Verification items for this drawing (mm, ordinates from the low corner). A direction names the side the tool comes from. Coordinates: 2 decimals unless noted, no trailing zeros. Write each loop counter-clockwise with the first axis right and the second up, starting at its lowest first coordinate (ties: lowest second). Pieces come first, ordered by that corner, then holes. Notation, with made-up numbers: (-7.5, 54) -> (51.5, 54) arc R15 cw to (51.5, 61) -> close; hole circle Ø7 at (74.25, 14). An arc over 180 degrees is marked (long way). One line per question, with ' | ' between items.
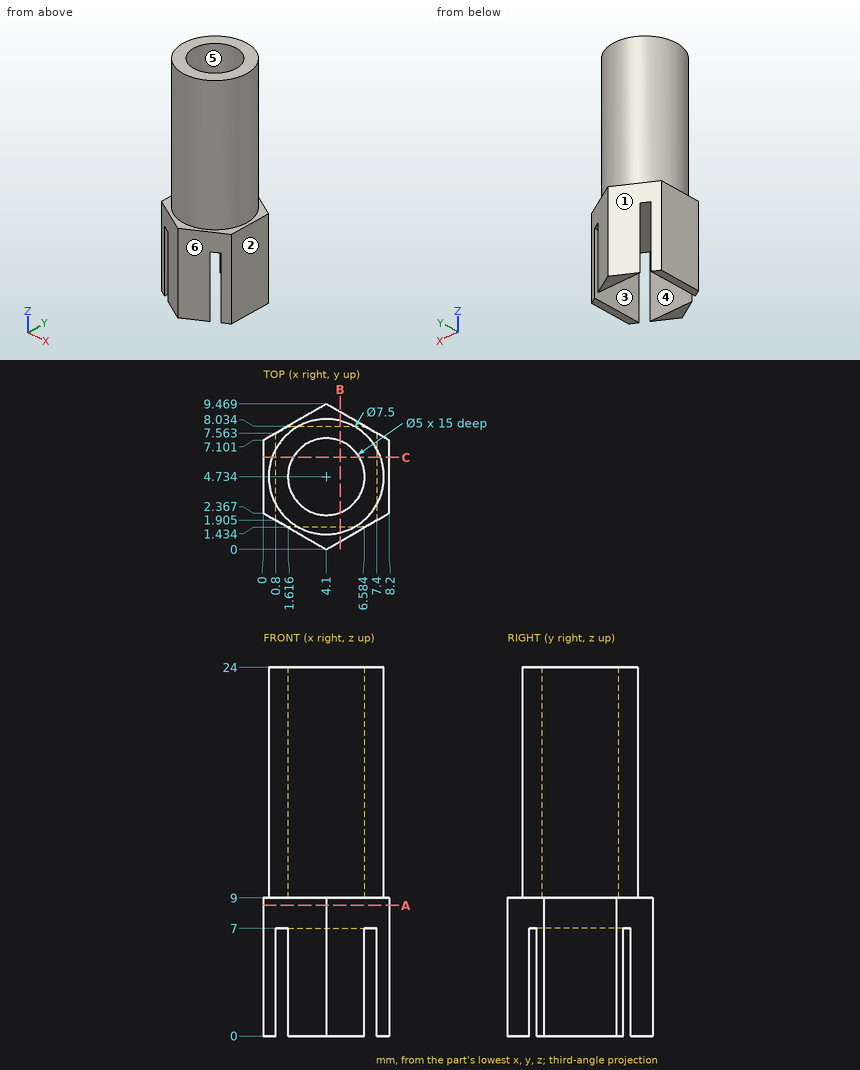
(1) Depth check by flat-ended pin: P1, Ø4, axis at y = 5.5, z = 11.5, coming from the +X side; P2, Ø1, axis at x = 5.5, y = 4, coming from the +Z side; P3, Ø3, axis at y = 8.5, z = 20, coming from the -X side; P4, Ø4, axis at x = 3, z = 4.5, coming from the +Y side. Enter the tip coordinate at first touch or a pass-through.
Answers below:
P1: stops at x = 7.85 | P2: stops at z = 9 | P3: stops at x = 1.11 | P4: stops at y = 9.47
(2) Material ranges on line 1 (Y direction, x = 4.1, z = 16) (1 decimal); line 2 (X direction, y = 4.75, z = 5.25); line 3 (Z direction, x = 4.5, y = 4.5), recorded low to high.
Answers below:
line 1: y = 1 to 2.2, 7.2 to 8.5 | line 2: x = 0 to 0.8, 7.4 to 8.2 | line 3: z = 7 to 9
(3) Cross-section at C-C (y = 6). Record the cut outline in (x, z) (1 decimal).
Answers below:
outline: (0, 0) -> (0.8, 0) -> (0.8, 7) -> (7.4, 7) -> (7.4, 0) -> (8.2, 0) -> (8.2, 9) -> (7.6, 9) -> (7.6, 24) -> (6.3, 24) -> (6.3, 9) -> (1.9, 9) -> (1.9, 24) -> (0.6, 24) -> (0.6, 9) -> (0, 9) -> close
(4) Cross-section at A-A (z = 8.5). Record the cut outline in (x, y).
Answers below:
outline: (0, 2.37) -> (4.1, 0) -> (8.2, 2.37) -> (8.2, 7.1) -> (4.1, 9.47) -> (0, 7.1) -> close
(5) Cross-section at B-B (x = 5). Record the cut outline in (y, z) (1 decimal).
Answers below:
outline: (0.5, 0) -> (1.4, 0) -> (1.4, 7) -> (8, 7) -> (8, 0) -> (8.9, 0) -> (8.9, 9) -> (8.4, 9) -> (8.4, 24) -> (7.1, 24) -> (7.1, 9) -> (2.4, 9) -> (2.4, 24) -> (1.1, 24) -> (1.1, 9) -> (0.5, 9) -> close
(6) Tool access check on the marked faces 4, 5 and 6. Record the directions out of +Z, -Z, +X, -X, +Y, -Y that give a thin tool (end or side, any length) a straight path to the whole face; none if there is none.
Answers below:
face 4: -Z, +X, -X | face 5: +Z | face 6: +Z, -Z, +X, -Y
(7) Draft check along X on the marked faces 1, 2 and 3. Enter one of: pulls with the +X half, pulls with the -X half, needs draft (parallel to the pull), parting line crosses it, or undercut.
Answers below:
face 1: pulls with the -X half | face 2: pulls with the +X half | face 3: undercut
